Design review of the part built by this model. Coordinates are the model's own, in mm. Give positions to 0.01 mm unless a question says otherwise; leave off trailing zeros. Order: outer loops, then holes, each group sorted by start corner. A loop starts at its lowest first (then second) coordinate and runs counter-clockwise, first axis right, second up. Notation, with made-up numbers: (75, -6) -> (91, -6) arc R25 ccw to (91, 17) -> close; hole circle Ø9 at (-15.5, 57.25). An arc over 180 degrees is marked (long way). One line per item, written item: value.
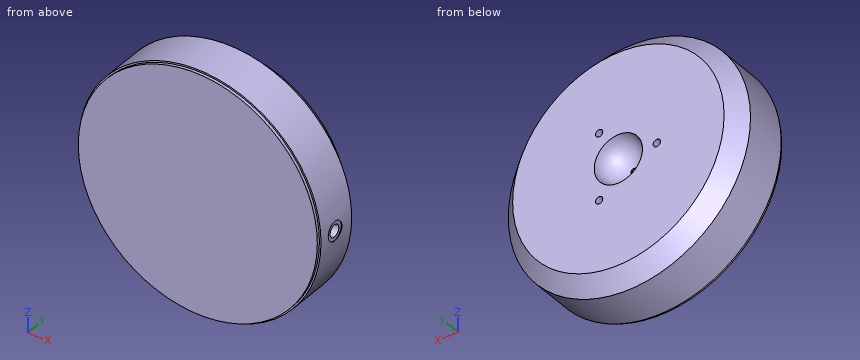
from build123d import *

# Parameters (mm, degrees)
M5X0_8_TAPPED_HOLE1_D                               = 4.2
M5X0_8_TAPPED_HOLE1_DEPTH                           = 46.99
M5X0_8_TAPPED_HOLE1_CBORE_D                         = 5
M5X0_8_TAPPED_HOLE1_CBORE_DEPTH                     = 7.62
M5X0_8_TAPPED_HOLE1_TIP                             = 1.2618073
CIRPATTERN1_COUNT                                   = 3
CBORE_FOR_00_BINDING_HEAD_MACHINE_SCREW_D           = 1.397
CBORE_FOR_00_BINDING_HEAD_MACHINE_SCREW_DEPTH       = 6.35
CBORE_FOR_00_BINDING_HEAD_MACHINE_SCREW_CBORE_D     = 7.874
CBORE_FOR_00_BINDING_HEAD_MACHINE_SCREW_CBORE_DEPTH = 0.254
CBORE_FOR_00_BINDING_HEAD_MACHINE_SCREW_TIP         = 0.419701142
SKETCH2_R                                           = 49.3395
EXTRUDE1_DEPTH                                      = 1.2192


with BuildPart() as part:
    # Sketch1 → Revolve1 (revolve)
    with BuildSketch(Plane.XY, mode=Mode.PRIVATE) as revolve1_sk:
        with BuildLine():
            Line((0, 0), (49.9999, 0))
            Line((49.9999, 0), (49.9999, 17.6276))
            Line((49.9999, 17.6276), (43.6499, 23.9776))
            Line((43.6499, 23.9776), (9.955892816, 23.9776))
            ThreePointArc((9.955892816, 23.9776), (7.139407653, 17.980689326), (1.1938, 15.057458932))
            Line((1.1938, 15.057458932), (1.1938, 14.5796))
            Line((1.1938, 14.5796), (0, 14.5796))
            Line((0, 14.5796), (0, 0))
        make_face()
    revolve(revolve1_sk.sketch.rotate(Axis((0, 23.9776, 0), (0, -1, 0)), 180), axis=Axis((0, 23.9776, 0), (0, -1, 0)))  # turned: the seam where the file's is

    # M5x0.8 Tapped Hole1
    with Locations(Plane(origin=(49.9999, 8.0772, 0), x_dir=(0, 0, 1), z_dir=(1, 0, 0))):
        with Locations((0, 0)):
            CounterBoreHole(M5X0_8_TAPPED_HOLE1_D / 2, M5X0_8_TAPPED_HOLE1_CBORE_D / 2, M5X0_8_TAPPED_HOLE1_CBORE_DEPTH, depth=M5X0_8_TAPPED_HOLE1_DEPTH)
            with Locations((0, 0, -(M5X0_8_TAPPED_HOLE1_DEPTH + M5X0_8_TAPPED_HOLE1_TIP / 2))):  # 118° drill point
                Cone(0, M5X0_8_TAPPED_HOLE1_D / 2, M5X0_8_TAPPED_HOLE1_TIP, mode=Mode.SUBTRACT)

    # Sketch5 → M3x0.5 Tapped Hole1 (revolve, cut)
    with BuildSketch(Plane(origin=(-15.875, 23.9776, 0), x_dir=(0, 0, 1), z_dir=(1, 0, 0))):
        Polygon((0, 0), (0, 10.403075774), (1.25, 9.652), (1.25, 5.9944), (1.5, 5.9944), (1.5, 0), align=None)
    m3x0_5_tapped_hole1 = revolve(axis=Axis((-15.875, 30.3276, 0), (0, -1, 0)), mode=Mode.SUBTRACT)

    # CirPattern1: M3x0.5 Tapped Hole1 ×3 about axis
    cirpattern1_axis = Axis((0, 0, 0), (0, 1, 0))
    for i in range(1, CIRPATTERN1_COUNT):
        add(m3x0_5_tapped_hole1.rotate(cirpattern1_axis, i * 360 / CIRPATTERN1_COUNT), mode=Mode.SUBTRACT)

    # CBORE for #00 Binding Head Machine Screw1
    with Locations(Plane(origin=(49.9999, 8.0772, 0), x_dir=(0, 0, 1), z_dir=(1, 0, 0))):
        with Locations((0, 0)):
            CounterBoreHole(CBORE_FOR_00_BINDING_HEAD_MACHINE_SCREW_D / 2, CBORE_FOR_00_BINDING_HEAD_MACHINE_SCREW_CBORE_D / 2, CBORE_FOR_00_BINDING_HEAD_MACHINE_SCREW_CBORE_DEPTH, depth=CBORE_FOR_00_BINDING_HEAD_MACHINE_SCREW_DEPTH)
            with Locations((0, 0, -(CBORE_FOR_00_BINDING_HEAD_MACHINE_SCREW_DEPTH + CBORE_FOR_00_BINDING_HEAD_MACHINE_SCREW_TIP / 2))):  # 118° drill point
                Cone(0, CBORE_FOR_00_BINDING_HEAD_MACHINE_SCREW_D / 2, CBORE_FOR_00_BINDING_HEAD_MACHINE_SCREW_TIP, mode=Mode.SUBTRACT)

    # Sketch2 → Extrude1 (add)
    with BuildSketch(Plane.XZ):
        with Locations(Location((0, 0, 0), (0, 0, 180))):  # turned: the seam where the file's is
            Circle(SKETCH2_R)
    extrude(amount=EXTRUDE1_DEPTH)


solid = part.part
Item 1: Add section C-C on y = 1.75. Give the boundary of the cut face in (x, z), plus the area to 3 significant figures.
Returned:
outline: circle Ø100 at (0, 0)
area: 7,850 mm²
Item 2: Add section B-B on y = 20.75. Give the boundary of the cut face in (x, z) (1 decimal), plus the area to 3 significant figures.
Returned:
outline: circle Ø93.8 at (0, 0); hole circle Ø3 at (-15.9, 0); hole circle Ø18.1 at (0, 0); hole circle Ø3 at (7.9, -13.7); hole circle Ø3 at (7.9, 13.7)
area: 6,620 mm²
Item 3: To check wall thickness, follow line 1 along Z through (x, y) = (-14.5, 21.75); line 2 along Y through (x, z) = (45, 0); line 3 along X through (y, z) = (21.5, -5). State the ranges of each line that lie inside material, in increasing order. Write a range as from..to.
Returned:
line 1: -43.53..-0.6, 0.6..43.53
line 2: -1.22..5.58, 10.58..22.63
line 3: -45.86..-7.93, 7.93..45.86
Item 4: Clearance check with flat-ended pins moving along their axes: P1, Ø0.7, axis at x = 0, z = 0, coming from the +Y side; P2, Ø12, axis at x = -36, y = 12, coming from the +Z side; P3, Ø1.5, axis at x = -15.875, z = 0, coming from the +Y side. State where each tip first meets the part, or that it passes through.
Returned:
P1: y = 14.58
P2: z = 40
P3: y = 14.03
Item 5: Add section A-A on x = 0. Give the boundary of the cut face in (y, z).
Returned:
outline: (-1.22, -49.34) -> (0, -49.34) -> (0, -50) -> (17.63, -50) -> (23.98, -43.65) -> (23.98, -9.96) arc R10.01 cw to (15.06, -1.19) -> (14.58, -1.19) -> (14.58, 1.19) -> (15.06, 1.19) arc R10.01 cw to (23.98, 9.96) -> (23.98, 43.65) -> (17.63, 50) -> (0, 50) -> (0, 49.34) -> (-1.22, 49.34) -> close
